Autodesk Inventor part; units mm, degrees
ref_plane "YZ Plane" through (0, 0, 0) normal (1, 0, 0) x (0, 1, 0)
ref_plane "XZ Plane" through (0, 0, 0) normal (0, 1, 0) x (-1, 0, 0)
ref_plane "XY Plane" through (0, 0, 0) normal (0, 0, 1) x (1, 0, 0)
sketch "Sketch1" plane through (0, 0, 0) normal (0, 0, 1) x (1, 0, 0)
  line L0 (0, 0) -> (25.4, 0)
  line L1 (25.4, 0) -> (25.4, 25.4)
  line L2 (25.4, 25.4) -> (0, 25.4)
  line L3 (0, 25.4) -> (0, 0)
  line L4 (3.175, 22.225) -> (22.225, 22.225)
  line L5 (22.225, 22.225) -> (22.225, 3.175)
  line L6 (22.225, 3.175) -> (3.175, 3.175)
  line L7 (3.175, 3.175) -> (3.175, 22.225)
  dimension "d0" = 25.4
  dimension "d1" = 25.4
  dimension "d2" = 3.175
extrude "Extrusion1" add sketch "Sketch1" against normal blind 114.3
sketch "Sketch2" plane through (0, 0, 0) normal (-1, 0, 0) x (0, 0, 1)
  line L0 (-114.3, 25.4) -> (-114.3, 0)
  point P0 (-101.6, 12.7)
  point P1 (-76.2, 12.7)
  point P2 (-50.8, 12.7)
  dimension "d5" = 12.7
  dimension "d6" = 25.4
  dimension "d7" = 25.4
hole "Hole1" at (0, 12.7, -101.6) at (0, 12.7, -76.2) at (0, 12.7, -50.8) direction (1, 0, 0) diameter 6.35 depth 25.4 tip angle 118
sketch "Sketch3" plane through (0, 0, 0) normal (0, -1, 0) x (1, 0, 0)
  line L0 (0, 0) -> (25.4, 0)
  point P0 (12.7, -12.7)
  dimension "d15" = 12.7
hole "Hole2" at (12.7, 0, -12.7) direction (0, 1, 0) diameter 6.35 depth 25.4 tip angle 118
properties part number "towerside4.5inbrace"
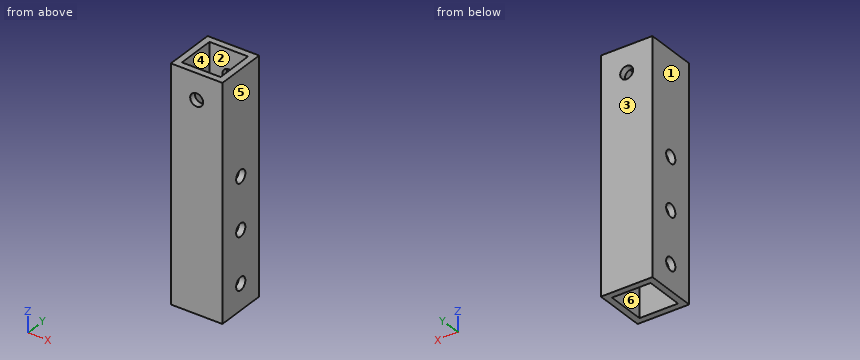
Could you check a few things on this model? Use its own coordinates, in mm. Face numbers are marked on the shaded views. A direction names the side the tool comes from. Round coordinates to 2 decimals unless told otherwise and drop trailing zeros. Loops run counter-clockwise (first coordinate to the right, second up) from the corner with the lowest first, then second, coordinate; pieces in that order, holes last. Notation, with made-up numbers: (70, 3) - (83, 3) arc R24 cw to (83, 25) - close; hole circle Ø4 at (15.25, 27). An arc over 180 degrees is marked (long way). Answer in a Markdown table with one row per item. Add a question column.
(1) For the marked faces 1 and 2, which set-ups out of +Z, -Z, +X, -X, +Y, -Y let a thin tool reach every point of the face, with its end or its side?
(2) If we section it at A-A (z = -12.7): Please give me the cut outline in (x, y) (3 decimals), plus the area to 3 significant figures.
(3) I need wall thicknesses on line 1 along Z through (x, y) = (1.2, 12.7) (3 decimals); line 2 along Y through (x, z) = (1, -101.6) (3 decimals); line 3 along X through (y, z) = (12, -57.5) (3 decimals). Which ranges of each line are inside material? Lowest first, please.
(4) If we section it at B-B (x = 12.7): Please give me the cut outline in (y, z) (3 decimals), plus the area to 3 significant figures.
(5) If we section it at C-C (y = 6.25): Please give me the cut outline in (x, z) (3 decimals), plus the area to 3 significant figures.
(6) If we mould it in two halves opening along Y, with no side actions, what happens to the marked faces 3, 4, 5 and 6? For each: pulls with the +Y half, pulls with the -Y half, needs draft (parallel to the pull), parting line crosses it, or undercut.
(7) If we section it at D-D (z = -28): Please give me the cut outline in (x, y) (3 decimals).
Model answer:
| question | item | result |
|---|---|---|
| 1 | face 1 | +Z, -Z, -X, +Y, -Y |
| 1 | face 2 | +Z, -Z |
| 2 | outline | (0, 0) - (9.525, 0) - (9.525, 3.175) - (3.175, 3.175) - (3.175, 22.225) - (9.525, 22.225) - (9.525, 25.4) - (0, 25.4) - close; (15.875, 0) - (25.4, 0) - (25.4, 25.4) - (15.875, 25.4) - (15.875, 22.225) - (22.225, 22.225) - (22.225, 3.175) - (15.875, 3.175) - close |
| 2 | area | 242 mm² |
| 3 | line 1 | z = -114.3 to -104.775, -98.425 to -79.375, -73.025 to -53.975, -47.625 to 0 |
| 3 | line 2 | y = 0 to 9.525, 15.875 to 25.4 |
| 3 | line 3 | x = 0 to 3.175, 22.225 to 25.4 |
| 4 | outline | (0, -114.3) - (3.175, -114.3) - (3.175, -15.875) - (0, -15.875) - close; (0, -9.525) - (3.175, -9.525) - (3.175, 0) - (0, 0) - close; (22.225, -114.3) - (25.4, -114.3) - (25.4, -15.875) - (22.225, -15.875) - close; (22.225, -9.525) - (25.4, -9.525) - (25.4, 0) - (22.225, 0) - close |
| 4 | area | 685 mm² |
| 5 | outline | (0, -114.3) - (3.175, -114.3) - (3.175, 0) - (0, 0) - close; (22.225, -114.3) - (25.4, -114.3) - (25.4, 0) - (22.225, 0) - close |
| 5 | area | 726 mm² |
| 6 | face 3 | pulls with the +Y half |
| 6 | face 4 | undercut |
| 6 | face 5 | needs draft |
| 6 | face 6 | undercut |
| 7 | outline | (0, 0) - (25.4, 0) - (25.4, 25.4) - (0, 25.4) - close; hole (3.175, 3.175) - (22.225, 3.175) - (22.225, 22.225) - (3.175, 22.225) - close |
